Study the drawing (mm; zero at the part's minimum x, y, z) and answer. A direction names the side the tool comes from. Coordinates: 2 decimals unless noted, no trailing zeros. Order: outer loops, then holes, each group sorted by start corner. A loop starts at its lowest first (then second) coordinate and runs counter-clockwise, first axis right, second up. Notation, with made-up numbers: (29, -26) -> (58, -26) arc R13 ccw to (58, -10) -> close; hole circle Ø2 at (79.5, 40). An arc over 180 degrees is marked (long way). Put each result on its own line as item: value. Start each with the question number.
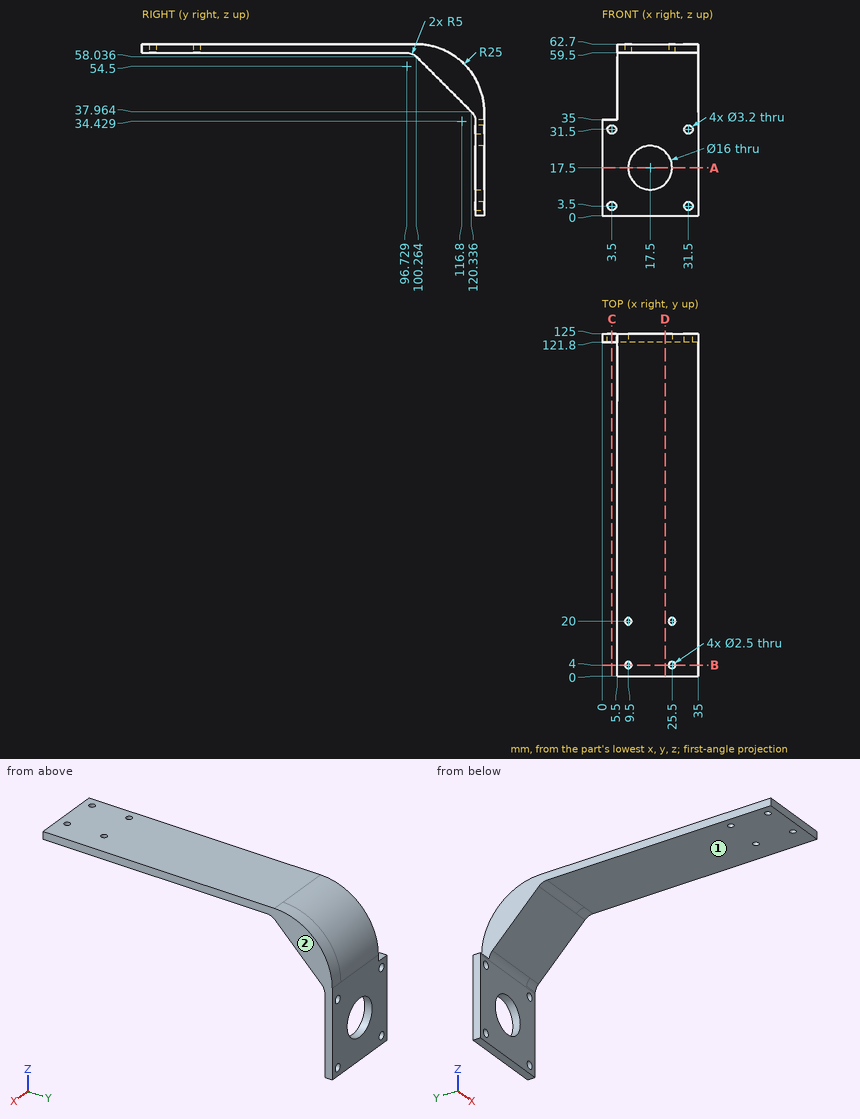
(1) The part is cut by section D-D on x = 23. Determine the outline of the cut face in (y, z) (1 decimal).
(2) The part is cut by section B-B on y = 4. Determine the outline of the cut face in (x, z).
(3) Find the intervals of material crossed by L1, parallel to X at y = 123.65, z = 3.5; L2, parallel to X at y = 122.85, z = 17.5; L3, parallel to X at y = 122, z = 3, in increasing order.
(4) The part is cut by section C-C on x = 3.5. Determine the outline of the cut face in (y, z).
(5) Each of these flat-tipped pins is pushed along its axis until it touches: P1, Ø2.5, axis at x = 3.5, y = 123.5, coming from the +Z side; P2, Ø9, axis at x = 15.5, y = 45, coming from the -Z side; P3, Ø6, axis at x = 21, z = 49.5, coming from the -Y side. Where does it stop, or does it pass through?
(6) A tool of negligible diameter and unlimited length cuts with its end or side. For the marked faces 1 and 2, from which of +Z, -Z, +X, -X, +Y, -Y can it reach the whole face along a straight path? Write none if from no direction.
(7) The part is cut by section A-A on z = 17.5. Determine the outline of the cut face in (x, y).
Worked out:
1. outline: (0, 59.5) -> (96.7, 59.5) arc R5 cw to (100.3, 58) -> (120.3, 38) arc R5 cw to (121.8, 34.4) -> (121.8, 23.3) -> (125, 23.3) -> (125, 37.7) arc R25 ccw to (100, 62.7) -> (0, 62.7) -> close; (121.8, 0) -> (125, 0) -> (125, 11.7) -> (121.8, 11.7) -> close
2. outline: (5.5, 59.5) -> (8.25, 59.5) -> (8.25, 62.7) -> (5.5, 62.7) -> close; (10.75, 59.5) -> (24.25, 59.5) -> (24.25, 62.7) -> (10.75, 62.7) -> close; (26.75, 59.5) -> (35, 59.5) -> (35, 62.7) -> (26.75, 62.7) -> close
3. L1: 0 to 1.9, 5.1 to 29.9, 33.1 to 35
3. L2: 0 to 9.5, 25.5 to 35
3. L3: 0 to 1.98, 5.02 to 29.98, 33.02 to 35
4. outline: (121.77, 35) arc R5 cw to (121.8, 34.43) -> (121.8, 33.1) -> (125, 33.1) -> (125, 35) -> close; (121.8, 0) -> (125, 0) -> (125, 1.9) -> (121.8, 1.9) -> close; (121.8, 5.1) -> (125, 5.1) -> (125, 29.9) -> (121.8, 29.9) -> close
5. P1: z = 35
5. P2: z = 59.5
5. P3: y = 105.8
6. face 1: -Z, +X, -X, -Y
6. face 2: +Z, -Z, +X, +Y, -Y
7. outline: (0, 121.8) -> (9.5, 121.8) -> (9.5, 125) -> (0, 125) -> close; (25.5, 121.8) -> (35, 121.8) -> (35, 125) -> (25.5, 125) -> close
